from build123d import *

# Parameters (mm, degrees)
ESQUISSE1_W             = 53.975
ESQUISSE1_H             = 12.7
BOSS_EXTRU_1_DEPTH      = 3.175
ESQUISSE2_R             = 2.032
ENL_V_MAT_EXTRU_1_DEPTH = 3.175
ESQUISSE3_W             = 53.975
ESQUISSE3_H             = 7.9375
BOSS_EXTRU_2_DEPTH      = 3.175
ESQUISSE4_W             = 53.975
ESQUISSE4_H             = 3.175
BOSS_EXTRU_3_DEPTH      = 12.7
ESQUISSE5_R             = 2.38125
ENL_V_MAT_EXTRU_2_DEPTH = 12.7
ESQUISSE6_W             = 18.084193737
ESQUISSE6_H             = 12.254267232
ESQUISSE6_W_2           = 18.044331553
ENL_V_MAT_EXTRU_3_DEPTH = 12.7
CONG_2_R                = 2.54


with BuildPart() as part:
    # Esquisse1 → Boss.-Extru.1 (new body)
    with BuildSketch(Plane(origin=(0, 0, 0), x_dir=(1, 0, 0), z_dir=(0, 1, 0))):
        with Locations((26.9875, 6.35)):
            Rectangle(ESQUISSE1_W, ESQUISSE1_H)
    extrude(amount=BOSS_EXTRU_1_DEPTH)

    # Esquisse2 → Enlèv. mat.-Extru.1 (cut)
    with BuildSketch(Plane(origin=(0, 3.175, 0), x_dir=(1, 0, 0), z_dir=(0, 1, 0))):
        with Locations(Location((4.826, 7.62, 0), (0, 0, 270))):
            Circle(ESQUISSE2_R)
        with Locations(Location((49.022, 7.62, 0), (0, 0, 270))):
            Circle(ESQUISSE2_R)
    extrude(amount=-ENL_V_MAT_EXTRU_1_DEPTH, mode=Mode.SUBTRACT)

    # Esquisse3 → Boss.-Extru.2 (add)
    with BuildSketch(Plane(origin=(0, 3.175, 0), x_dir=(1, 0, 0), z_dir=(0, 1, 0))):
        with Locations((26.9875, -3.96875)):
            Rectangle(ESQUISSE3_W, ESQUISSE3_H)
    extrude(amount=-BOSS_EXTRU_2_DEPTH)

    # Esquisse4 → Boss.-Extru.3 (add)
    with BuildSketch(Plane(origin=(0, 3.175, 0), x_dir=(1, 0, 0), z_dir=(0, 1, 0))):
        with Locations((26.9875, -6.35)):
            Rectangle(ESQUISSE4_W, ESQUISSE4_H)
    extrude(amount=BOSS_EXTRU_3_DEPTH)

    # Esquisse5 → Enlèv. mat.-Extru.2 (cut)
    with BuildSketch(Plane.XY.offset(7.9375)):
        with Locations((21.844, 12.7)):
            Circle(ESQUISSE5_R)
        with Locations((32.16275, 12.7)):
            Circle(ESQUISSE5_R)
    extrude(amount=-ENL_V_MAT_EXTRU_2_DEPTH, mode=Mode.SUBTRACT)

    # Esquisse6 → Enlèv. mat.-Extru.3 (cut)
    with BuildSketch(Plane.XY.offset(7.9375)):
        with Locations((9.042096868, 9.747866384)):
            Rectangle(ESQUISSE6_W, ESQUISSE6_H)
        with Locations((44.952834224, 9.747866384)):
            Rectangle(ESQUISSE6_W_2, ESQUISSE6_H)
    extrude(amount=-ENL_V_MAT_EXTRU_3_DEPTH, mode=Mode.SUBTRACT)

    # Congé2
    cong_2_edges = [part.edges().sort_by_distance(p)[0] for p in [
        (26.9875, 0, 7.9375),
        (26.9875, 0, -12.7),
        (53.975, 0, -2.38125),
        (0, 0, -2.38125),
        (35.930668447, 15.875, 6.35),
        (18.084193737, 15.875, 6.35),
    ]]
    fillet(cong_2_edges, radius=CONG_2_R)


solid = part.part
Geometry: final body of the model. Coordinates: model frame, mm. A direction names the side the tool comes from. Give positions to 0.01 mm unless a question says otherwise; leave off trailing zeros. Write each loop counter-clockwise with the first axis right and the second up, starting at its lowest first coordinate (ties: lowest second). Pieces come first, ordered by that corner, then holes.
(1) Cut plane B-B, the plane z = -7.62. Return loops of the section in (x, y) (3 decimals).
(2) Cut plane C-C, the plane x = 50.5. Return loops of the section in (y, z) (1 decimal), then the cut area to 3 significant figures.
(3) Mould query, pull axis X, two halves, no side actions, for faces 1 (the flat face through (27, 0, -2)), 2 (the flat face through (53.975, 3, -2)), 3 (the cylindrical face through (51.037, 1.61, -7.885)), 4 (the cylindrical face through (19.465, 12.805, 6.372)). Classes: released by +X, released by -X, zero draft, split by the parting line, or undercut.
(4) Access query for faces 5 (the flat face through (9, 3.621, 6)), 6 (the flat face through (27, 3.175, -4)), 7 (the flat face through (0, 3, -2)), 8 (the cylindrical face through (4.92, 1.61, -9.65)), 9 (the flat face through (35.931, 8, 6)). Directions: +Z, -Z, +X, -X, +Y, -Y. A direction counts if a zero-diameter tool reaches every point of the face in a straight line with its end or side. Return the directions, or none.
(5) First-contact query: P1, Ø6.5, axis at x = 30.5, y = 9.5, coming from the -Z side; P2, Ø2, axis at x = 28.5, z = -4.5, coming from the +Y side (3 decimals); P3, Ø3.5, axis at x = 8.5, z = 7, coming from the +Y side; P4, Ø4, axis at x = 21.844, y = 12.7, coming from the +Z side. Flat tips, straight axial feed; report the tip coordinate or a pass-through.
(6) Cut plane A-A, the plane y = 12.7. Return loops of the section in (x, z).
(7) Ray query, line 1 (Y direction, x = 43, z = 3) (3 decimals); line 2 (Y direction, x = 14, z = -11.25) (3 decimals); line 3 (Z direction, x = 19, y = 10.5). Return the intervals inside material, ascending.
(8) Cut plane D-D, the plane x = 44. Return loops of the section in (y, z) (1 decimal), then the cut area to 3 significant figures.
Values follow:
1. outline: (0, 2.54) arc R2.54 ccw to (2.54, 0) - (2.794, 0) - (2.794, 3.175) - (0, 3.175) - close; (6.858, 0) - (46.99, 0) - (46.99, 3.175) - (6.858, 3.175) - close; (51.054, 0) - (51.435, 0) arc R2.54 ccw to (53.975, 2.54) - (53.975, 3.175) - (51.054, 3.175) - close
2. outline: (0, -10.2) arc R2.5 ccw to (2.5, -12.7) - (3.2, -12.7) - (3.2, -9) - (0, -9) - close; (0, -6.2) - (3.2, -6.2) - (3.2, 4.8) - (3.6, 4.8) - (3.6, 7.9) - (2.5, 7.9) arc R2.5 ccw to (0, 5.4) - close
2. area: 55.3 mm2
3. face 1: zero draft
3. face 2: released by +X
3. face 3: undercut
3. face 4: undercut
4. face 5: +Z, -Z, -X, +Y
4. face 6: -Z, +X, -X, +Y
4. face 7: +Z, -Z, -X, +Y, -Y
4. face 8: +Y, -Y
4. face 9: +Z, -Z, +X, +Y
5. P1: stops at z = 4.76
5. P2: stops at y = 3.175
5. P3: stops at y = 3.62
5. P4: passes through
6. outline: (18.08, 4.76) - (19.46, 4.76) - (19.46, 7.94) - (18.08, 7.94) - close; (24.23, 4.76) - (29.78, 4.76) - (29.78, 7.94) - (24.23, 7.94) - close; (34.54, 4.76) - (35.93, 4.76) - (35.93, 7.94) - (34.54, 7.94) - close
7. line 1: y = 0 to 3.175
7. line 2: y = 0.246 to 3.175
7. line 3: z = 4.76 to 7.94
8. outline: (0, -10.2) arc R2.5 ccw to (2.5, -12.7) - (3.2, -12.7) - (3.2, 4.8) - (3.6, 4.8) - (3.6, 7.9) - (2.5, 7.9) arc R2.5 ccw to (0, 5.4) - close
8. area: 64.2 mm2
